from build123d import *

# Parameters (mm, degrees)
SKETCH1_W           = 6.35
SKETCH1_H           = 22.225
BOSS_EXTRUDE1_DEPTH = 3.175


with BuildPart() as part:
    # Sketch1 → Boss-Extrude1 (new, symmetric)
    with BuildSketch(Plane.XY):
        Rectangle(SKETCH1_W, SKETCH1_H)
        with BuildLine():
            Line((-1.5, -7.9375), (-1.5, 7.9375))
            ThreePointArc((-1.5, 7.9375), (0, 9.4375), (1.5, 7.9375))
            Line((1.5, 7.9375), (1.5, -7.9375))
            ThreePointArc((1.5, -7.9375), (0, -9.4375), (-1.5, -7.9375))
        make_face(mode=Mode.SUBTRACT)
    extrude(amount=BOSS_EXTRUDE1_DEPTH, both=True)


solid = part.part
Read the model definition and answer for the solid it produces. Units are mm, in the model's axes. A direction names the side the tool comes from. Coordinates: 2 decimals unless noted, no trailing zeros. Loops run counter-clockwise (first coordinate to the right, second up) from the corner with the lowest first, then second, coordinate; pieces in that order, holes last.
Q1. The part is cut by section A-A on x = 0. Write down the section's boundary in (y, z) (1 decimal), and give its area (3 significant figures).
Q2. The part is cut by section B-B on y = -5. Write down the section's boundary in (x, z) (3 decimals).
Q3. This flat-tipped pin is pushed along its axis until it touches: pin 1 Ø3 at (x, y) = (0.5, -1.5) entering from +Z (3 decimals). Where does it stop, or does it pass through?
Q4. Consider probe 1 along X at (y, z) = (-1.5, -1.5) (3 decimals); probe 2 along X at (y, z) = (9.25, -2.25) (3 decimals); probe 3 along Y at (x, z) = (-1.25, 2.75). Determine where each line is inside the solid, lowest interval first.
Q5. The part is cut by section C-C on z = 2.75. Write down the section's boundary in (x, y) (1 decimal).
Q6. The mould has two halves that part along Y. Classify faces 3 (the face through (0, 11.112, 0)), 4 (the face through (0, -11.112, 0)), 5 (the face through (-3.175, 0, 0)), 6 (the face through (-1.5, 0, 0)): +Y half, -Y half, draft (parallel to the pull), parting line (faces both ways), or undercut.
Q7. Which of the six approach directions +Z, -Z, +X, -X, +Y, -Y give full straight-line access (tool end or side, diameter ignored) to faces 1 (the face through (-0.033, 9.437, 0.044)), 2 (the face through (3.175, 0, 0))?
Results below:
1. outline: (-11.1, -3.2) - (-9.4, -3.2) - (-9.4, 3.2) - (-11.1, 3.2) - close; (9.4, -3.2) - (11.1, -3.2) - (11.1, 3.2) - (9.4, 3.2) - close
1. area: 21.3 mm2
2. outline: (-3.175, -3.175) - (-1.5, -3.175) - (-1.5, 3.175) - (-3.175, 3.175) - close; (1.5, -3.175) - (3.175, -3.175) - (3.175, 3.175) - (1.5, 3.175) - close
3. pin 1: stops at z = 3.175
4. probe 1: x = -3.175 to -1.5, 1.5 to 3.175
4. probe 2: x = -3.175 to -0.726, 0.726 to 3.175
4. probe 3: y = -11.11 to -8.77, 8.77 to 11.11
5. outline: (-3.2, -11.1) - (3.2, -11.1) - (3.2, 11.1) - (-3.2, 11.1) - close; hole (-1.5, -7.9) arc R1.5 ccw to (1.5, -7.9) - (1.5, 7.9) arc R1.5 ccw to (-1.5, 7.9) - close
6. face 3: +Y half
6. face 4: -Y half
6. face 5: draft
6. face 6: undercut
7. face 1: +Z, -Z
7. face 2: +Z, -Z, +X, +Y, -Y
